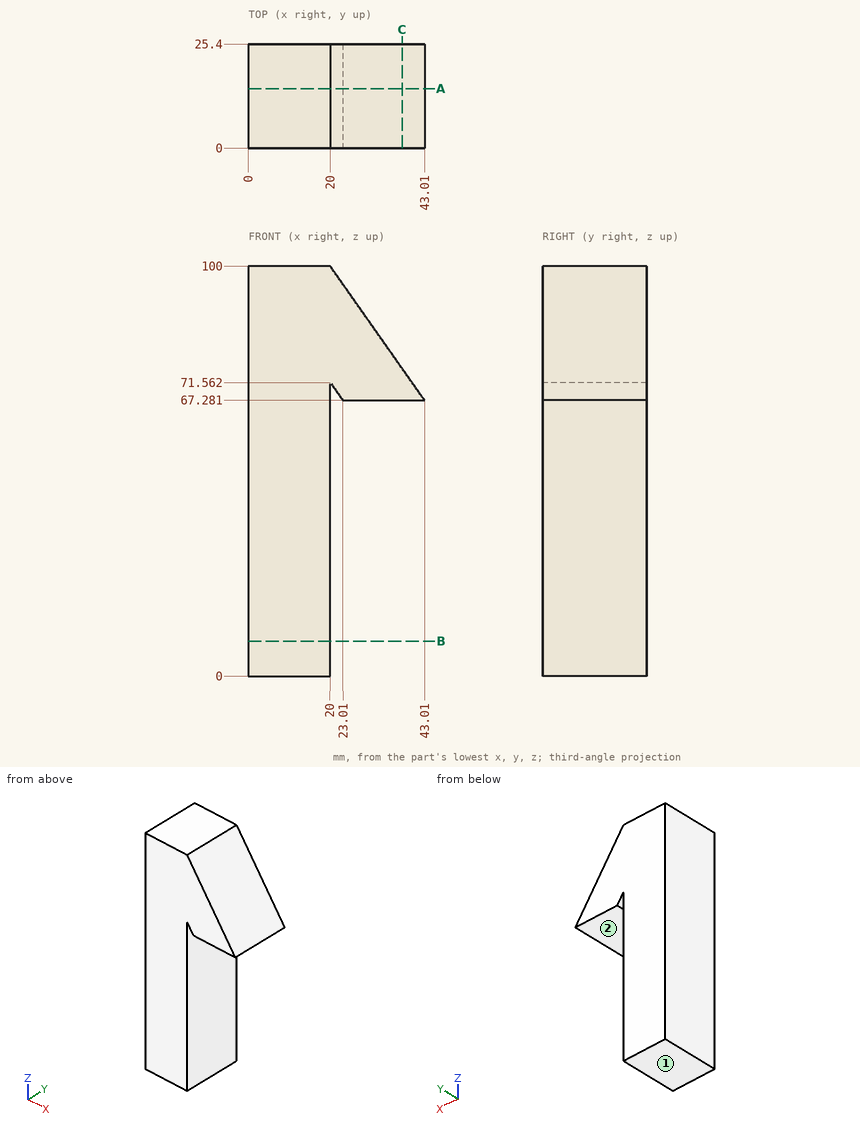
The figure shows three views and two pictorial views of one solid part (mm, origin at its lowest corner). Answer the questions. A direction names the side the tool comes from. Coordinates: 2 decimals unless noted, no trailing zeros. Loops run counter-clockwise (first coordinate to the right, second up) from the corner with the lowest first, then second, coordinate; pieces in that order, holes last. Notation, with made-up numbers: (85, 56) - (128, 56) arc R22 ccw to (128, 95) - close; hole circle Ø11 at (87, 66.5). An arc over 180 degrees is marked (long way). Answer in a Markdown table with one row per item.
Q1. Straight lines are drawn through the part: line 1 along X through (y, z) = (16.5, 54); line 2 along Z through (x, y) = (28.5, 21.5) (1 decimal); line 3 along X through (y, z) = (17.75, 91.5). For each, find the intervals that lie inside material, in ascending order. Write a range as [from, to].
Here are the results:
| item | result |
|---|---|
| line 1 | x = [0, 20] |
| line 2 | z = [67.3, 87.9] |
| line 3 | x = [0, 25.98] |
Q2. Find section C-C on x = 37.5. Write down the section's boundary in (y, z).
Here are the results:
| item | result |
|---|---|
| outline | (0, 67.28) - (25.4, 67.28) - (25.4, 75.12) - (0, 75.12) - close |
Q3. Find section A-A on y = 14.5. Write down the section's boundary in (x, z).
Here are the results:
| item | result |
|---|---|
| outline | (0, 0) - (20, 0) - (20, 71.56) - (23.01, 67.28) - (43.01, 67.28) - (20, 100) - (0, 100) - close |
Q4. Given P1, Ø2, axis at y = 4.5, z = 78.5, coming from the +X side; P2, Ø1.5, axis at x = 29, y = 11, coming from the -Z side; P3, Ø12.5, axis at y = 17.5, z = 20, coming from the +X side, each flat-ended and moving along its own axis, determine where each tip first touches the part or whether it passes through.
Here are the results:
| item | result |
|---|---|
| P1 | stops at x = 35.82 |
| P2 | stops at z = 67.28 |
| P3 | stops at x = 20 |
Q5. For the marked faces 1 and 2, determine the directions among +Z, -Z, +X, -X, +Y, -Y from which every point of the face is accessible in a straight line to the end or side of a thin tool.
Here are the results:
| item | result |
|---|---|
| face 1 | -Z, +X, -X, +Y, -Y |
| face 2 | -Z, +X, +Y, -Y |
Q6. Find section B-B on z = 8.5. Write down the section's boundary in (x, y).
Here are the results:
| item | result |
|---|---|
| outline | (0, 0) - (20, 0) - (20, 25.4) - (0, 25.4) - close |
